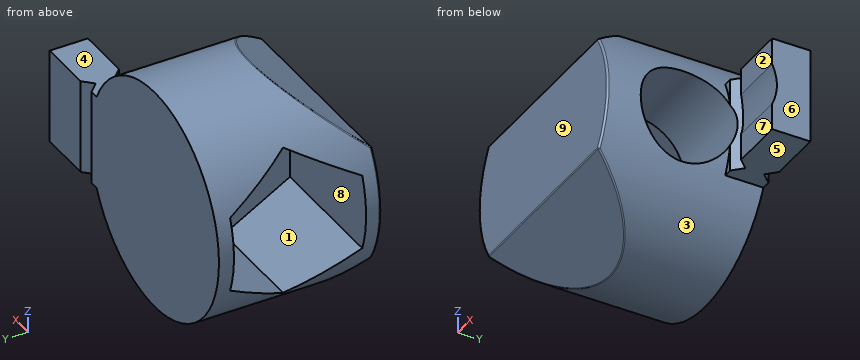
from build123d import *

# Parameters (mm, degrees)
SKETCH1_R          = 5.9
EXTRUDE1_DEPTH     = 8.5
SKETCH2_W          = 9.65
SKETCH2_H          = 5
EXTRUDE2_DEPTH     = 2
SKETCH3_R          = 2.5
CUT_EXTRUDE1_DEPTH = 16.55
CUT_EXTRUDE2_DEPTH = 9.4000001
CUT_EXTRUDE3_DEPTH = 16.5500001
FILLET2_R          = 0.1
CUT_EXTRUDE5_DEPTH = 7


with BuildPart() as part:
    # Sketch1 → Extrude1 (new body)
    with BuildSketch(Plane(origin=(0, 0, 0), x_dir=(1, 0, 0), z_dir=(0, 1, 0))):
        Circle(SKETCH1_R)
    extrude(amount=EXTRUDE1_DEPTH)

    # Sketch2 → Extrude2 (add)
    with BuildSketch(Plane(origin=(0, 8.5, 0), x_dir=(1, 0, 0), z_dir=(0, 1, 0))):
        with Locations((4.825, 0)):
            Rectangle(SKETCH2_W, SKETCH2_H)
    extrude(amount=-EXTRUDE2_DEPTH)

    # Sketch3 → Cut-Extrude1 (cut, through all)
    with BuildSketch(Plane(origin=(9.65, 0, 0), x_dir=(0, 0, -1), z_dir=(1, 0, 0))):
        with Locations((0, 4.25)):
            Circle(SKETCH3_R)
    extrude(amount=-CUT_EXTRUDE1_DEPTH, mode=Mode.SUBTRACT)

    # Sketch4 → Cut-Extrude2 (cut, through all)
    with BuildSketch(Plane.XY.offset(2.5)):
        Polygon((6.8, 8.5), (5.8, 8.5), (6.3, 8), align=None)
        Polygon((6.3, 7), (5.8, 6.5), (6.8, 6.5), align=None)
    extrude(amount=-CUT_EXTRUDE2_DEPTH, mode=Mode.SUBTRACT)

    # Sketch5 → Cut-Extrude3 (cut, through all)
    with BuildSketch(Plane(origin=(9.65, 0, 0), x_dir=(0, 0, -1), z_dir=(1, 0, 0))):
        Polygon((-5.9, 3.5), (-6.106265144, 3.5), (-6.003132572, -0.278643129), (6.106265144, -0.15610938), (6.106265144, 3.632225684), (5.9, 3.5), (3, 0), (-3, 0), align=None)
    extrude(amount=-CUT_EXTRUDE3_DEPTH, mode=Mode.SUBTRACT)

    # Fillet2
    fillet2_edges = [part.edges().sort_by_distance(p)[0] for p in [
        (5.691400991, 0, -1.554977415),
        (-5.9, 0, 0),
        (0, 0, -3),
        (0, 0, 3),
        (-3.201105027, 2.360810271, 4.956099939),
        (3.201105027, 2.360810271, -4.956099939),
    ]]
    fillet(fillet2_edges, radius=FILLET2_R)

    # Sketch7 → Cut-Extrude5 (cut)
    with BuildSketch(Plane(origin=(-5.9, 0, 0), x_dir=(0, 0, -1), z_dir=(1, 0, 0))):
        Polygon((-4, 4.25), (-2, 7.714101615), (2, 7.714101615), (4, 4.25), (2, 0.785898385), (-2, 0.785898385), align=None)
    extrude(amount=CUT_EXTRUDE5_DEPTH, mode=Mode.SUBTRACT)


solid = part.part
Design review of the part built by this model. Coordinates are the model's own, in mm. Face numbers are marked on the shaded views. A direction names the side the tool comes from. Coordinates: 2 decimals unless noted, no trailing zeros. Write each loop counter-clockwise with the first axis right and the second up, starting at its lowest first coordinate (ties: lowest second). Pieces come first, ordered by that corner, then holes. Notation, with made-up numbers: (82, 56.25) - (127, 56.25) arc R30 ccw to (127, 85.25) - close; hole circle Ø4 at (12.25, -6). An arc over 180 degrees is marked (long way). One line per item, written item: value.
1) Mouldability with a two-part tool opening along Z and no side actions: class the marked faces 1, 2, 3 and 4 as +Z half, -Z half, draft (parallel to the pull), parting line (faces both ways), or undercut.
Answer sheet:
face 1: undercut
face 2: draft
face 3: parting line
face 4: +Z half
2) For the marked faces 5, 6, 7, 8 and 9, list the 3-axis set-ups (+Z, -Z, +X, -X, +Y, -Y) from which the entire face can be reached by the end or side of a thin tool; tool diameter is ignored.
Answer sheet:
face 5: -Z, +X, +Y, -Y
face 6: +Z, -Z, +X, +Y, -Y
face 7: +Z, -Z, +X, -Y
face 8: -X
face 9: +Z, -Z, +X, -X, -Y
3) Add section A-A (z = 0). State the section outline as (x, y) points.
Answer sheet:
outline: (-5.9, 0.1) arc R0.1 ccw to (-5.8, 0) - (5.8, 0) arc R0.1 ccw to (5.9, 0.1) - (5.9, 1.75) - (1.1, 1.75) - (1.1, 0.79) - (-5.9, 0.79) - close; (-5.9, 7.71) - (1.1, 7.71) - (1.1, 6.75) - (6.05, 6.75) - (6.3, 7) - (6.55, 6.75) - (9.65, 6.75) - (9.65, 8.5) - (6.8, 8.5) - (6.3, 8) - (5.8, 8.5) - (-5.9, 8.5) - close
4) Add section C-C (y = 7.5). State the section outline as (x, z) points, plus the area to 3 significant figures.
Answer sheet:
outline: (-5.5, -2.12) arc R5.9 ccw to (5.34, -2.5) - (9.65, -2.5) - (9.65, 2.5) - (5.34, 2.5) arc R5.9 ccw to (-5.5, 2.12) - (1.1, 2.12) - (1.1, -2.12) - close
area: 99.8 mm2
5) Insertion check: pin 1 (1.5 mm diameter, centred on x = 5, y = 7, fed in from +Z); pin 2 (2 mm diameter, centred on x = 7, y = 7.5, fed in from -Z); pin 3 (2 mm diameter, centred on x = 8, y = 7.5, fed in from +Z). Each pin has a flat end and moves straight along its axis. Give the tip position at first contact, or say it passes through.
Answer sheet:
pin 1: stops at z = 4.09
pin 2: stops at z = -2.5
pin 3: stops at z = 2.5
6) Add section B-B (y = 5.25). State the section outline as (x, z) points, plus the area to 3 significant figures.
Answer sheet:
outline: (-4.81, -3.42) arc R5.9 ccw to (5.44, -2.29) - (1.1, -2.29) - (1.1, -3.42) - close; (-4.81, 3.42) - (1.1, 3.42) - (1.1, 2.29) - (5.44, 2.29) arc R5.9 ccw to start
area: 42.5 mm2
7) To check wall thickness, follow probe 1 along Y at (x, z) = (2.35, 0); probe 2 along Y at (x, z) = (-4, -0.25); probe 3 along Z at (x, y) = (4.15, 4.25). State the ranges of each line that lie inside material, in increasing order.
Answer sheet:
probe 1: y = 0 to 1.75, 6.75 to 8.5
probe 2: y = 0 to 0.79, 7.71 to 8.5
probe 3: z = -4.19 to -2.5, 2.5 to 4.19
